from build123d import *
from build123d.topology import SkipClean

# Parameters (mm, degrees)
ESQUISSE1_R                                = 30
BOSS_EXTRU_1_DEPTH                         = 15
ESQUISSE2_R                                = 12.5
BOSS_EXTRU_2_DEPTH                         = 184
ESQUISSE4_2_W                              = 230
ESQUISSE4_2_H                              = 40
ENL_V_MAT_EXTRU_1_DEPTH                    = 5
CHAMBRAGE_POUR_VIS_T_TE_HEXAGONALE_2_COUNT = 2
CHAMBRAGE_POUR_VIS_T_TE_HEXAGONALE_2_PITCH = 41
ESQUISSE17_R                               = 6
BOSS_EXTRU_4_DEPTH                         = 83.38
ESQUISSE18_W                               = 10.356322474
ESQUISSE18_H                               = 3
ENL_V_MAT_EXTRU_2_DEPTH                    = 3
ESQUISSE19_W                               = 7.933443835
ESQUISSE19_H                               = 21.9317122
ENL_V_MAT_EXTRU_3_DEPTH                    = 50
BOSS_EXTRU_6_START                         = -10
ESQUISSE21_R                               = 12.5
BOSS_EXTRU_6_DEPTH                         = 10
ESQUISSE26_R                               = 17.5
BOSS_EXTRU_8_DEPTH                         = 112
ENL_V_START                                = -92
ESQUISSE27_R                               = 17.5
ENL_V_MAT_EXTRU_5_DEPTH                    = 92
ENL_V_START_2                              = -15
ESQUISSE28_R                               = 30
ENL_V_MAT_EXTRU_6_DEPTH                    = 15
BOSS_EXTRU_9_START                         = 10
BOSS_EXTRU_9_DEPTH                         = 10
D_GAGEMENT_M61_D                           = 6.6
D_GAGEMENT_M61_DEPTH                       = 4
D_GAGEMENT_M61_TIP                         = 1.905255888


with BuildPart() as part:
    # Esquisse1 → Boss.-Extru.1 (new body)
    with BuildSketch(Plane.XY):
        Circle(ESQUISSE1_R)
    extrude(amount=BOSS_EXTRU_1_DEPTH)

    # Esquisse2 → Boss.-Extru.2 (add)
    with BuildSketch(Plane(origin=(0, 0, 0), x_dir=(-1, 0, 0), z_dir=(0, 0, -1))):
        with Locations(Location((0, 0, 0), (0, 0, 180))):
            Circle(ESQUISSE2_R)
    extrude(amount=BOSS_EXTRU_2_DEPTH)

    # Esquisse4_2 → Enl_v. mat.-Extru.1 (cut)
    with BuildSketch(Plane.XY.offset(15)):
        Rectangle(ESQUISSE4_2_W, ESQUISSE4_2_H)
    extrude(amount=-ENL_V_MAT_EXTRU_1_DEPTH, mode=Mode.SUBTRACT)

    # Esquisse14 → Chambrage pour vis _ t_te hexagonale M51 (revolve, cut)
    with BuildSketch(Plane.YZ.offset(-20.5)):
        Polygon((0, 0), (0, 15), (2.75, 15), (2.75, 3.605), (2.775, 3.58), (6.12, 3.58), (6.12, 0), align=None)
    chambrage_pour_vis_t_te_hexagonale_m51 = revolve(axis=Axis((-20.5, 0, -6.35), (0, 0, 1)), mode=Mode.SUBTRACT)

    # Chambrage pour vis _ t_te hexagonale 2: Chambrage pour vis _ t_te hexagonale M51 ×2
    with Locations(*[(i * CHAMBRAGE_POUR_VIS_T_TE_HEXAGONALE_2_PITCH, 0, 0) for i in range(1, CHAMBRAGE_POUR_VIS_T_TE_HEXAGONALE_2_COUNT)]):
        add(chambrage_pour_vis_t_te_hexagonale_m51, mode=Mode.SUBTRACT)

    # Esquisse17 → Boss.-Extru.4 (add)
    with BuildSketch(Plane(origin=(0, 0, -184), x_dir=(-1, 0, 0), z_dir=(0, 0, -1))):
        Circle(ESQUISSE17_R)
    extrude(amount=BOSS_EXTRU_4_DEPTH)

    # Esquisse18 → Enl_v. mat.-Extru.2 (cut)
    with BuildSketch(Plane(origin=(0, 0, -267.38), x_dir=(-1, 0, 0), z_dir=(0, 0, -1))):
        with Locations((1.787207702, 0)):
            Rectangle(ESQUISSE18_W, ESQUISSE18_H)
    extrude(amount=-ENL_V_MAT_EXTRU_2_DEPTH, mode=Mode.SUBTRACT)

    # Esquisse19 → Enl_v. mat.-Extru.3 (cut)
    with BuildSketch(Plane(origin=(0, 0, -184), x_dir=(-1, 0, 0), z_dir=(0, 0, -1))):
        with Locations((9.966721917, 0)):
            Rectangle(ESQUISSE19_W, ESQUISSE19_H)
    extrude(amount=-ENL_V_MAT_EXTRU_3_DEPTH, mode=Mode.SUBTRACT)

    # Esquisse21 → Boss.-Extru.6 (add)
    with BuildSketch(Plane(origin=(0, 0, -184), x_dir=(-1, 0, 0), z_dir=(0, 0, -1)).offset(BOSS_EXTRU_6_START)):
        with Locations(Location((0, 0, 0), (0, 0, 180))):
            Circle(ESQUISSE21_R)
    extrude(amount=BOSS_EXTRU_6_DEPTH)

    # Esquisse26 → Boss.-Extru.8 (add)
    with BuildSketch(Plane(origin=(0, 0, -134), x_dir=(-1, 0, 0), z_dir=(0, 0, -1))):
        Circle(ESQUISSE26_R)
    extrude(amount=-BOSS_EXTRU_8_DEPTH)

    # Esquisse27 → Enl_v. mat.-Extru.5 (cut)
    with SkipClean():  # the faces are left unmerged after this step: merging them gives an invalid solid
        with BuildSketch(Plane(origin=(0, 0, -134), x_dir=(-1, 0, 0), z_dir=(0, 0, -1)).offset(ENL_V_START)):
            Circle(ESQUISSE27_R)
            with BuildLine():
                ThreePointArc((6, 10.9658561), (10.752906584, 6.373774392), (12.5, 0))
                ThreePointArc((12.5, 0), (10.752906584, -6.373774392), (6, -10.9658561))
                ThreePointArc((6, -10.9658561), (-12.5, 0), (6, 10.9658561))
            make_face(mode=Mode.SUBTRACT)
        extrude(amount=ENL_V_MAT_EXTRU_5_DEPTH, mode=Mode.SUBTRACT)

    # Esquisse28 → Enl_v. mat.-Extru.6 (cut)
    with SkipClean():  # the faces are left unmerged after this step: merging them gives an invalid solid
        with BuildSketch(Plane.XY.offset(15).offset(ENL_V_START_2)):
            Circle(ESQUISSE28_R)
        extrude(amount=ENL_V_MAT_EXTRU_6_DEPTH, mode=Mode.SUBTRACT)

    # Esquisse29 → Boss.-Extru.9 (add)
    with SkipClean():  # the faces are left unmerged after this step: merging them gives an invalid solid
        with BuildSketch(Plane.XY.offset(BOSS_EXTRU_9_START)):
            with BuildLine():
                Line((-4, -11.842719282), (-4, -8.5))
                Line((-4, -8.5), (4, -8.5))
                Line((4, -8.5), (4, -11.842719282))
                ThreePointArc((4, -11.842719282), (10.155048006, -7.288689869), (12.5, 0))
                ThreePointArc((12.5, 0), (-7.288689869, 10.155048006), (-4, -11.842719282))
            make_face()
        extrude(amount=-BOSS_EXTRU_9_DEPTH)

    # D_gagement M61
    with Locations(Plane.XY.offset(10)):
        with Locations((0, 0)):
            Hole(D_GAGEMENT_M61_D / 2, depth=D_GAGEMENT_M61_DEPTH)
            with Locations((0, 0, -(D_GAGEMENT_M61_DEPTH + D_GAGEMENT_M61_TIP / 2))):  # 120° drill point
                Cone(0, D_GAGEMENT_M61_D / 2, D_GAGEMENT_M61_TIP, mode=Mode.SUBTRACT)


solid = part.part
Source: CAD feature listing. Evaluate the final solid. Frame: model axes, mm. A direction names the side the tool comes from. Round coordinates to 2 decimals unless told otherwise and drop trailing zeros. Loops run counter-clockwise (first coordinate to the right, second up) from the corner with the lowest first, then second, coordinate; pieces in that order, holes last.
Q1. First-contact query: P1, Ø3.5, axis at x = -2, z = -265, coming from the -Y side; P2, Ø1.5, axis at x = -8.5, y = 12, coming from the +Z side; P3, Ø2.5, axis at y = -10, z = 7, coming from the -X side. Flat tips, straight axial feed; report the tip coordinate or a pass-through.
Q2. Section C-C, the plane x = 9.5. Return loops of the section in (y, z), plus the area to 3 significant figures.
Q3. Section D-D, the plane z = -222. Return loops of the section in (x, y), plus the area to 3 significant figures.
Q4. Section A-A, the plane x = -10. Return loops of the section in (y, z).
Q5. Ray query, line 1 (Y direction, x = 0, z = 8.6); line 2 (Z direction, x = -10.5, y = 6); line 3 (Z direction, x = 7, y = 4). Return the intervals inside material, ascending.
Q6. Access query for faces 1 (the face through (-8, 0, -134)), 2 (the face through (5.4, -3, -184)), 3 (the face through (0, -8.5, 5)), 4 (the face through (-8, -11, -22)). Directions: +Z, -Z, +X, -X, +Y, -Y. A direction counts if a zero-diameter tool reaches every point of the face in a straight line with its end or side. Return the directions, or none.
Q7. Mould query, pull axis Y, two halves, no side actions, for faces 5 (the face through (13.887, -10.648, -32.14)), 6 (the face through (3, 3, 10)), 7 (the face through (-0.124, -0.559, 4.426)), 8 (the face through (2.43, 2.23, 7.97)). Classes: pulls with the +Y half, pulls with the -Y half, needs draft (parallel to the pull), parting line crosses it, or undercut.
Q8. Section B-B, the plane z = -116. Return loops of the section in (x, y), plus the area to 3 significant figures.
Solutions:
1. P1: stops at y = -5.99
1. P2: stops at z = -22
1. P3: stops at x = -8.93
2. outline: (-14.7, -42) - (-8.12, -42) - (-8.12, -184) - (8.12, -184) - (8.12, -42) - (14.7, -42) - (14.7, -22) - (8.12, -22) - (8.12, 10) - (-8.12, 10) - (-8.12, -22) - (-14.7, -22) - close
2. area: 3,420 mm2
3. outline: circle Ø12 at (0, 0)
3. area: 113 mm2
4. outline: (-14.36, -42) - (-7.5, -42) - (-7.5, -134) - (7.5, -134) - (7.5, -42) - (14.36, -42) - (14.36, -22) - (7.5, -22) - (7.5, 10) - (-7.5, 10) - (-7.5, -22) - (-14.36, -22) - close; (-7.5, -184) - (7.5, -184) - (7.5, -174) - (-7.5, -174) - close
5. line 1: y = -8.5 to -3.3, 3.3 to 12.5
5. line 2: z = -184 to -174, -134 to 10
5. line 3: z = -184 to 10
6. face 1: -X, +Y, -Y
6. face 2: -Z
6. face 3: +Z, -Y
6. face 4: +Z
7. face 5: parting line crosses it
7. face 6: needs draft
7. face 7: undercut
7. face 8: undercut
8. outline: circle Ø25 at (0, 0)
8. area: 491 mm2
